Can you work these out from the drawing? Everything is in mm from the part's minimum corner. A direction names the side the tool comes from. Round coordinates to 2 decimals unless told otherwise and drop trailing zeros. Loops run counter-clockwise (first coordinate to the right, second up) from the corner with the lowest first, then second, coordinate; pieces in that order, holes last. Notation, with made-up numbers: (30.25, 29) -> (57.25, 29) arc R13 ccw to (57.25, 34) -> close; hole circle Ø11 at (-23, -7). An arc over 180 degrees is marked (long way). Answer as a JSON object with one key per item and string values.
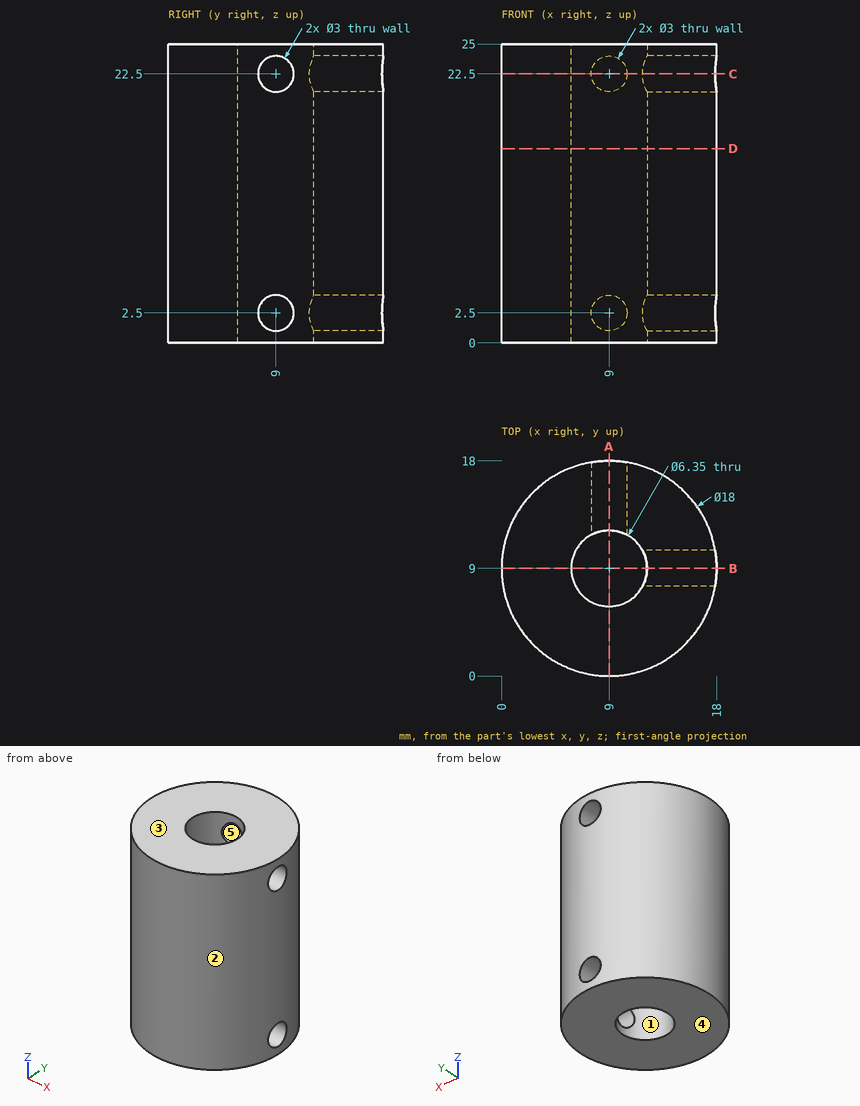
Q1. We'd pull the mould along Y, two halves only. Please class the marked faces 1, 2 and 3: pulls with the +Y half, pulls with the -Y half, needs draft (parallel to the pull), parting line crosses it, or undercut.
Determined:
{"face 1": "undercut", "face 2": "parting line crosses it", "face 3": "needs draft"}
Q2. On a 3-axis mill with a long thin cutter (end or side, diameter ignored), from which of +Z, -Z, +X, -X, +Y, -Y can I reach the whole of each face in a straight line? I mean the marked faces 4 and 5. Say none if no direction works.
Determined:
{"face 4": "-Z, +X, -X, +Y, -Y", "face 5": "+Y"}
Q3. If I drill on L1, parallel to Z at x = 9, y = 16.75; L2, parallel to Y at x = 9, z = 16.75 (3 decimals); L3, parallel to Z at x = 9.75, y = 14.25, over which ranges is the centre line in solid material (lowest first)? Write a range as [from, to].
Determined:
{"L1": "[0, 1], [4, 21], [24, 25]", "L2": "[0, 5.825], [12.175, 18]", "L3": "[0, 1.2], [3.8, 21.2], [23.8, 25]"}
Q4. I want a section at C-C, the plane z = 22.5. Write out the boundary of the cut face in (x, y) (3 decimals).
Determined:
{"outline": "(7.5, 11.798) -> (7.5, 17.874) arc R9 ccw (long way) to (17.874, 7.5) -> (11.798, 7.5) arc R3.175 cw (long way) to start; (10.5, 11.798) arc R3.175 cw to (11.798, 10.5) -> (17.874, 10.5) arc R9 ccw to (10.5, 17.874) -> close"}
Q5. I want a section at A-A, the plane x = 9. Write out the boundary of the cut face in (y, z) (3 decimals).
Determined:
{"outline": "(0, 0) -> (5.825, 0) -> (5.825, 25) -> (0, 25) -> close; (12.175, 0) -> (18, 0) -> (18, 1) -> (12.175, 1) -> close; (12.175, 4) -> (18, 4) -> (18, 21) -> (12.175, 21) -> close; (12.175, 24) -> (18, 24) -> (18, 25) -> (12.175, 25) -> close"}
Q6. I want a section at D-D, the plane z = 16.25. Write out the boundary of the cut face in (x, y) (3 decimals), then the cut area to 3 significant figures.
Determined:
{"outline": "circle Ø18 at (9, 9); hole circle Ø6.35 at (9, 9)", "area": "223 mm²"}
Q7. I'm going to push flat-ended pins straight in: pin 1 (6 mm diameter, centred on y = 16, z = 11.5, fed in from -X); pin 2 (2.5 mm diameter, centred on x = 9, z = 22.5, fed in from +Y). Where does each tip first touch, or does it pass through?
Determined:
{"pin 1": "x = 0.94", "pin 2": "y = 6.08"}
